Model file for the job. Use its own axes, mm. Coordinates: 2 decimals unless noted, no trailing zeros. Loops run counter-clockwise (first coordinate to the right, second up) from the corner with the lowest first, then second, coordinate; pieces in that order, holes last. Notation, with made-up numbers: (13, 5.5) -> (64, 5.5) arc R28 cw to (64, 41.5) -> close; hole circle Ø9 at (-2.75, 67.25). An arc over 180 degrees is marked (long way). Use one line per item in the form item = value.
```python
from build123d import *

# Parameters (mm, degrees)
SKETCH1_W           = 5
SKETCH1_H           = 25
BOSS_EXTRUDE1_DEPTH = 258.5
SKETCH2_R           = 3
SKETCH2_R_2         = 1.5
CUT_EXTRUDE1_DEPTH  = 259.850342862


with BuildPart() as part:
    # Sketch1 → Boss-Extrude1 (new body)
    with BuildSketch(Plane.XY):
        Rectangle(SKETCH1_W, SKETCH1_H)
    extrude(amount=BOSS_EXTRUDE1_DEPTH)

    # Sketch2 → Cut-Extrude1 (cut, through all)
    with BuildSketch(Plane(origin=(2.5, 0, 0), x_dir=(0, 0, -1), z_dir=(1, 0, 0))):
        with Locations((-12.5, 0)):
            Circle(SKETCH2_R)
        with Locations((-246, 0)):
            Circle(SKETCH2_R_2)
        with Locations((-228, 0)):
            Circle(SKETCH2_R_2)
        with Locations((-48.5, 0)):
            Circle(SKETCH2_R_2)
        with Locations((-31.5, 0)):
            Circle(SKETCH2_R_2)
        with Locations((-138.5, 0)):
            Circle(SKETCH2_R_2)
        with BuildLine():
            Line((-12.5, 12.5), (5.5, 12.5))
            Line((5.5, 12.5), (5.5, -12.5))
            Line((5.5, -12.5), (-12.5, -12.5))
            ThreePointArc((-12.5, -12.5), (0, 0), (-12.5, 12.5))
        make_face()
        Polygon((-257.716878365, 0), (-250.5, 12.5), (-258.5, 12.5), (-258.5, -12.5), (-250.5, -12.5), align=None)
    extrude(amount=-CUT_EXTRUDE1_DEPTH, mode=Mode.SUBTRACT)


solid = part.part
```
Q1. Band-saw the part on A-A, the plane x = -1.75. Write the cut outline in (y, z).
Result:
outline = (-12.5, 12.5) arc R12.5 ccw to (12.5, 12.5) -> (12.5, 250.5) -> (0, 257.72) -> (-12.5, 250.5) -> close; hole circle Ø6 at (0, 12.5); hole circle Ø3 at (0, 31.5); hole circle Ø3 at (0, 48.5); hole circle Ø3 at (0, 138.5); hole circle Ø3 at (0, 228); hole circle Ø3 at (0, 246)
Q2. Mould opens along Y. For faces 1 (the face through (0, -12.5, 130)), 2 (the face through (2.5, 0, 127)), 3 (the face through (0, -1.8, 14.9)) say: released by +Y, released by -Y, zero draft, split by the parting line, or undercut.
Result:
face_1 = released by -Y
face_2 = zero draft
face_3 = undercut
Q3. Pin check, flat tip, straight feed: pin 1 Ø2 at (x, y) = (-1.5, -4) entering from +Z. Stop position of the tip, or through.
Result:
pin_1 = 255.98
Q4. Band-saw the part on B-B, the plane y = -9.5. Write the cut outline in (x, z), and give its area (3 significant figures).
Result:
outline = (-2.5, 4.38) -> (2.5, 4.38) -> (2.5, 252.23) -> (-2.5, 252.23) -> close
area = 1,240 mm2
Q5. Wall check: line 1 along Y through (x, z) = (1.35, 48.5); line 2 along Z through (x, y) = (-1.1, 2.25); line 3 along Z through (x, y) = (-1.4, 2). Give the ranges that are in metal, low to high.
Result:
line_1 = -12.5 to -1.5, 1.5 to 12.5
line_2 = 0.2 to 10.52, 14.48 to 256.42
line_3 = 0.16 to 10.26, 14.74 to 256.56
